Work out the finished part from the listing and answer in its coordinate system (mm). Face numbers are marked on the shaded views. A direction names the side the tool comes from. Round coordinates to 2 decimals unless told otherwise and drop trailing zeros. Write each loop counter-clockwise with the first axis right and the second up, starting at its lowest first coordinate (ties: lowest second). Pieces come first, ordered by that corner, then holes. Notation, with made-up numbers: (59, 56.5) - (69, 56.5) arc R28 cw to (69, 74.5) - close; hole circle Ø10 at (-16.5, 28.5). An arc over 180 degrees is marked (long way). Answer as a JSON object with one key per item and string values.
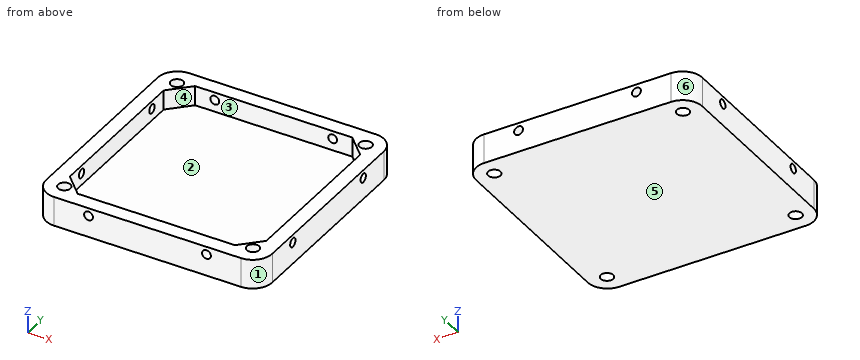
```python
from build123d import *

# Parameters (mm, degrees)
SKETCH1_W                                  = 115
SKETCH1_H                                  = 115
BOSS_EXTRUDE1_DEPTH                        = 7.5
FILLET1_R                                  = 10
SKETCH2_W                                  = 100
SKETCH2_H                                  = 100
CUT_EXTRUDE1_DEPTH                         = 10
CHAMFER1_SIZE                              = 10
SKETCH3_R                                  = 3.15
CUT_EXTRUDE2_DEPTH                         = 30
MIRROR1_AT_THE_SECOND_PLANE_COPY_1_SKETC_R = 3.15
MIRROR1_AT_THE_SECOND_PLANE_COPY_1_DEPTH   = 30
SKETCH4_R                                  = 2.25
CUT_EXTRUDE3_DEPTH                         = 130
SKETCH6_R                                  = 2.25
CUT_EXTRUDE4_DEPTH                         = 129.792468724


with BuildPart() as part:
    # Sketch1 → Boss-Extrude1 (new, symmetric)
    with BuildSketch(Plane.XY):
        Rectangle(SKETCH1_W, SKETCH1_H)
    extrude(amount=BOSS_EXTRUDE1_DEPTH, both=True)

    # Fillet1
    fillet1_edges = [part.edges().sort_by_distance(p)[0] for p in [
        (-57.5, 57.5, 0),
        (57.5, 57.5, 0),
        (57.5, -57.5, 0),
        (-57.5, -57.5, 0),
    ]]
    fillet(fillet1_edges, radius=FILLET1_R)

    # Sketch2 → Cut-Extrude1 (cut)
    with BuildSketch(Plane.XY.offset(7.5)):
        Rectangle(SKETCH2_W, SKETCH2_H)
    extrude(amount=-CUT_EXTRUDE1_DEPTH, mode=Mode.SUBTRACT)

    # Chamfer1
    chamfer1_edges = [part.edges().sort_by_distance(p)[0] for p in [
        (-50, -50, 2.5),
        (-50, 50, 2.5),
        (50, 50, 2.5),
        (50, -50, 2.5),
    ]]
    chamfer(chamfer1_edges, length=CHAMFER1_SIZE)

    # Sketch3 → Cut-Extrude2 (cut)
    with BuildSketch(Plane.XY.offset(7.5)):
        with Locations((-48, 48)):
            Circle(SKETCH3_R)
    cut_extrude2 = extrude(amount=-CUT_EXTRUDE2_DEPTH, mode=Mode.SUBTRACT)

    # Mirror1: Cut-Extrude2 across plane
    add(cut_extrude2.mirror(Plane(origin=(0, 0, 0), x_dir=(0, 0, 1), z_dir=(1, 0, 0))), mode=Mode.SUBTRACT)

    # Mirror1 at the second plane: Cut-Extrude2 across plane
    add(cut_extrude2.mirror(Plane.ZX), mode=Mode.SUBTRACT)

    # Mirror1 at the second plane copy 1 sketc → Mirror1 at the second plane copy 1 (cut)
    with BuildSketch(Plane(origin=(0, 0, 7.5), x_dir=(-1, 0, 0), z_dir=(0, 0, 1))):
        with Locations((-48, 48)):
            Circle(MIRROR1_AT_THE_SECOND_PLANE_COPY_1_SKETC_R)
    extrude(amount=-MIRROR1_AT_THE_SECOND_PLANE_COPY_1_DEPTH, mode=Mode.SUBTRACT)

    # Sketch4 → Cut-Extrude3 (cut)
    with BuildSketch(Plane(origin=(57.5, 0, 0), x_dir=(0, 0, -1), z_dir=(1, 0, 0))):
        with Locations((-3.5, 30)):
            Circle(SKETCH4_R)
    cut_extrude3 = extrude(amount=-CUT_EXTRUDE3_DEPTH, mode=Mode.SUBTRACT)

    # Mirror2: Cut-Extrude3 across plane
    add(cut_extrude3.mirror(Plane.ZX), mode=Mode.SUBTRACT)

    # Sketch6 → Cut-Extrude4 (cut, through all)
    with BuildSketch(Plane(origin=(0, 57.5, 0), x_dir=(1, 0, 0), z_dir=(0, 1, 0))):
        with Locations(Location((-30, -3.5, 0), (0, 0, 180))):
            Circle(SKETCH6_R)
    cut_extrude4 = extrude(amount=-CUT_EXTRUDE4_DEPTH, mode=Mode.SUBTRACT)

    # Mirror3: Cut-Extrude4 across plane
    add(cut_extrude4.mirror(Plane(origin=(0, 0, 0), x_dir=(0, 0, 1), z_dir=(1, 0, 0))), mode=Mode.SUBTRACT)


solid = part.part
```
Item 1: A cutting plane is placed at A-A (y = -30). Write down the section's boundary in (x, z), and give its area (4 significant figures).
Results found:
{"outline": "(-57.5, -7.5) - (57.5, -7.5) - (57.5, 1.25) - (50, 1.25) - (50, -2.5) - (-50, -2.5) - (-50, 1.25) - (-57.5, 1.25) - close; (-57.5, 5.75) - (-50, 5.75) - (-50, 7.5) - (-57.5, 7.5) - close; (50, 5.75) - (57.5, 5.75) - (57.5, 7.5) - (50, 7.5) - close", "area": "657.5 mm²"}
Item 2: A cutting plane is placed at D-D (z = 3.5). Give the number of separate pieces and of enclosed holes in the cut face, and give its area (3 significant figures).
Results found:
{"separate pieces": "8", "enclosed holes": "4", "area": "2,940 mm²"}
Item 3: Each of these flat-tipped pins is pushed along its axis until it touches: P1, Ø10, axis at x = 48, y = 48, coming from the -Z side; P2, Ø6, axis at x = 28.5, y = -44, coming from the +Z side. Where does it stop, or does it pass through?
Results found:
{"P1": "z = -7.5", "P2": "z = -2.5"}
Item 4: A cutting plane is placed at C-C (x = 14). Write down the section's boundary in (y, z), and give its area (3 significant figures).
Results found:
{"outline": "(-57.5, -7.5) - (57.5, -7.5) - (57.5, 7.5) - (50, 7.5) - (50, -2.5) - (-50, -2.5) - (-50, 7.5) - (-57.5, 7.5) - close", "area": "725 mm²"}
Item 5: Consider line 1 along Z through (x, y) = (-30, -56); line 2 along X through (y, z) = (28, 1.25). Determine where each line is inside the solid, lowest interval first.
Results found:
{"line 1": "-7.5 to 1.25, 5.75 to 7.5", "line 2": "-57.5 to -50, 50 to 57.5"}
Item 6: Determine the mould class of the marked faces 3, 4, 5 and 6 for opening direction X: pulls with the +X half, pulls with the -X half, needs draft (parallel to the pull), parting line crosses it, or undercut.
Results found:
{"face 3": "undercut", "face 4": "undercut", "face 5": "needs draft", "face 6": "pulls with the -X half"}
Item 7: For the marked faces 1 and 2, determine the directions among +Z, -Z, +X, -X, +Y, -Y from which every point of the face is accessible in a straight line to the end or side of a thin tool.
Results found:
{"face 1": "+Z, -Z, +X, -Y", "face 2": "+Z"}
